Can you work these out from the model? Positions are in its coordinate system, mm. A direction names the side the tool comes from. Give positions to 0.01 mm unless a question says otherwise; leave off trailing zeros. Order: outer loops, then holes, each group sorted by start corner. A loop starts at its lowest first (then second) coordinate and runs counter-clockwise, first axis right, second up. Notation, with made-up numbers: M 36,29 L 95,29 A17 ccw 95,51 Z; hole C 73,10 d2. An arc over 180 degrees is marked long. Use one line per item in the form item = value. Start each with the question number.
1. I want a section at B-B, the plane z = 67. List the corners of the cut face in (x, y) for me, and give its area (3 significant figures).
2. I need wall thicknesses on L1, parallel to Y at x = 4, z = 12; L2, parallel to Y at x = 4, z = 102.5; L3, parallel to Z at x = 22.5, y = 38. Which ranges of each line are inside material? Lowest first, please.
3. For faces 5 (the face through (0, -10, 58)), 6 (the face through (1.479, -7.876, 100.979)), 7 (the face through (-8, 2.96, 103)), which set-ups out of +Z, -Z, +X, -X, +Y, -Y let a thin tool reach every point of the face, with its end or its side?
4. I want a section at A-A, the plane y = 12. List the corners of the cut face in (x, z) for me.
5. Will these pins go through, and if not, where does the flat tip stop? P1, Ø10.5, axis at x = -8, z = 32, coming from the -Y side; P2, Ø2, axis at y = 8.5, z = 49, coming from the -X side; P3, Ø1, axis at y = -2, z = 34.5, coming from the -X side.
6. I want a section at C-C, the plane y = 60.21. List the corners of the cut face in (x, z) for me, and give its area (3 significant figures).
7. I want a section at D-D, the plane x = 14. List the corners of the cut face in (y, z) for me (3 decimals).
8. We'd pull the mould along Z, two halves only. Please class faces 1 (the face through (32.195, 61.697, 1.232)), 2 (the face through (1.48, -7.9, 11.02)), 3 (the face through (14, 24, 0)), 4 (the face through (14, 24, 115)): +Z half, -Z half, draft (parallel to the pull), parting line (faces both ways), or undercut.
```python
from build123d import *

# Parameters (mm, degrees)
SALIENTE_EXTRUIR1_DEPTH = 115
CROQUIS5_W              = 76.000174198
CROQUIS5_H              = 57.319794633
CORTAR_EXTRUIR2_DEPTH   = 16
CROQUIS6_W              = 76.000174198
CROQUIS6_H              = 7.5
CROQUIS6_W_2            = 76
SALIENTE_EXTRUIR2_DEPTH = 10.35
REDONDEO1_R             = 1
CROQUIS7_W              = 115
CROQUIS7_H              = 90
SALIENTE_EXTRUIR3_DEPTH = 5
CROQUIS14_W             = 115
CROQUIS14_H             = 90
CROQUIS14_W_2           = 110
CROQUIS14_H_2           = 85
SALIENTE_EXTRUIR5_DEPTH = 30
CORTAR_EXTRUIR5_REACH   = 26.29
CROQUIS15_R             = 1.8
CORTAR_EXTRUIR6_REACH   = 4.5
CORTAR_EXTRUIR7_DEPTH   = 3
CROQUIS19_R             = 1.5
CORTAR_EXTRUIR8_DEPTH   = 116


with BuildPart() as part:
    # Croquis1 → Saliente-Extruir1 (new body)
    with BuildSketch(Plane.XY):
        with BuildLine():
            Line((0, 49.71), (-16.64, 49.71))
            ThreePointArc((-16.64, 49.71), (-17.347106781, 49.417106781), (-17.64, 48.71))
            Line((-17.64, 48.71), (-17.64, 35.71))
            ThreePointArc((-17.64, 35.71), (-17.347106781, 35.002893219), (-16.64, 34.71))
            Line((-16.64, 34.71), (-16.322634469, 34.71))
            ThreePointArc((-16.322634469, 34.71), (-15.745851008, 34.89310292), (-15.380289019, 35.375358322))
            Line((-15.380289019, 35.375358322), (-14.64, 37.46))
            Line((-14.64, 37.46), (-13.64, 37.46))
            Line((-13.64, 37.46), (-13.64, 3.96))
            ThreePointArc((-13.64, 3.96), (-13.347106781, 3.252893219), (-12.64, 2.96))
            Line((-12.64, 2.96), (-4.22, 2.96))
            ThreePointArc((-4.22, 2.96), (-3.72, 2.46), (-4.22, 1.96))
            Line((-4.22, 1.96), (-14.72, 1.96))
            Line((-14.72, 1.96), (-14.72, 4.12))
            Line((-14.72, 4.12), (-14.839626167, 4.12))
            ThreePointArc((-14.839626167, 4.12), (-15.19514923, 4.054667509), (-15.504217878, 3.867206703))
            Line((-15.504217878, 3.867206703), (-18.954591711, 0.798323834))
            ThreePointArc((-18.954591711, 0.798323834), (-19.202302502, 0.460634096), (-19.29, 0.051117131))
            Line((-19.29, 0.051117131), (-19.29, 0))
            Line((-19.29, 0), (0, 0))
            Line((0, 0), (0, 49.71))
        make_face()
    extrude(amount=SALIENTE_EXTRUIR1_DEPTH)

    # Croquis5 → Cortar-Extruir2 (cut)
    with BuildSketch(Plane.ZY.offset(19.29)):
        with Locations((53, 24.620732186)):
            Rectangle(CROQUIS5_W, CROQUIS5_H)
    extrude(amount=-CORTAR_EXTRUIR2_DEPTH, mode=Mode.SUBTRACT)

    # Croquis6 → Saliente-Extruir2 (add)
    with BuildSketch(Plane.ZY.offset(3.29)):
        with Locations((53, 45.96)):
            Rectangle(CROQUIS6_W, CROQUIS6_H)
        with Locations((52.999912901, 6.71)):
            Rectangle(CROQUIS6_W_2, CROQUIS6_H)
    extrude(amount=SALIENTE_EXTRUIR2_DEPTH)

    # Redondeo1
    redondeo1_edges = [part.edges().sort_by_distance(p)[0] for p in [
        (-13.64, 2.96, 52.999912901),
    ]]
    fillet(redondeo1_edges, radius=REDONDEO1_R)

    # Croquis7 → Saliente-Extruir3 (add)
    with BuildSketch(Plane(origin=(0, 0, 0), x_dir=(0, 0, -1), z_dir=(1, 0, 0))):
        with Locations((-57.5, 24.71)):
            Rectangle(CROQUIS7_W, CROQUIS7_H)
    extrude(amount=SALIENTE_EXTRUIR3_DEPTH)

    # Croquis14 → Saliente-Extruir5 (add)
    with BuildSketch(Plane(origin=(5, 0, 0), x_dir=(0, 0, -1), z_dir=(1, 0, 0))):
        with Locations((-57.5, 24.71)):
            Rectangle(CROQUIS14_W, CROQUIS14_H)
        with Locations((-57.5, 24.71)):
            Rectangle(CROQUIS14_W_2, CROQUIS14_H_2, mode=Mode.SUBTRACT)
    extrude(amount=SALIENTE_EXTRUIR5_DEPTH)

    # Croquis15 → Cortar-Extruir5 (cut, up to next)
    with BuildSketch(Plane(origin=(5, 0, 0), x_dir=(0, 0, -1), z_dir=(1, 0, 0)), mode=Mode.PRIVATE) as cortar_extruir5_sk1:
        with Locations((-102.5, 54.71)):
            Circle(CROQUIS15_R)
    cortar_extruir5_tool1 = extrude(cortar_extruir5_sk1.sketch, amount=-CORTAR_EXTRUIR5_REACH, mode=Mode.PRIVATE) & part.part
    add(cortar_extruir5_tool1.solids().sort_by_distance((5, 54.71, 102.5))[0], mode=Mode.SUBTRACT)
    # Croquis15 → Cortar-Extruir5 (cut, up to next)
    with BuildSketch(Plane(origin=(5, 0, 0), x_dir=(0, 0, -1), z_dir=(1, 0, 0)), mode=Mode.PRIVATE) as cortar_extruir5_sk2:
        with Locations((-102.5, -5.29)):
            Circle(CROQUIS15_R)
    cortar_extruir5_tool2 = extrude(cortar_extruir5_sk2.sketch, amount=-CORTAR_EXTRUIR5_REACH, mode=Mode.PRIVATE) & part.part
    add(cortar_extruir5_tool2.solids().sort_by_distance((5, -5.29, 102.5))[0], mode=Mode.SUBTRACT)
    # Croquis15 → Cortar-Extruir5 (cut, up to next)
    with BuildSketch(Plane(origin=(5, 0, 0), x_dir=(0, 0, -1), z_dir=(1, 0, 0)), mode=Mode.PRIVATE) as cortar_extruir5_sk3:
        with Locations((-12.5, -5.29)):
            Circle(CROQUIS15_R)
    cortar_extruir5_tool3 = extrude(cortar_extruir5_sk3.sketch, amount=-CORTAR_EXTRUIR5_REACH, mode=Mode.PRIVATE) & part.part
    add(cortar_extruir5_tool3.solids().sort_by_distance((5, -5.29, 12.5))[0], mode=Mode.SUBTRACT)
    # Croquis15 → Cortar-Extruir5 (cut, up to next)
    with BuildSketch(Plane(origin=(5, 0, 0), x_dir=(0, 0, -1), z_dir=(1, 0, 0)), mode=Mode.PRIVATE) as cortar_extruir5_sk4:
        with Locations((-12.5, 54.71)):
            Circle(CROQUIS15_R)
    cortar_extruir5_tool4 = extrude(cortar_extruir5_sk4.sketch, amount=-CORTAR_EXTRUIR5_REACH, mode=Mode.PRIVATE) & part.part
    add(cortar_extruir5_tool4.solids().sort_by_distance((5, 54.71, 12.5))[0], mode=Mode.SUBTRACT)

    # Croquis16 → Cortar-Extruir6 (cut, up to next)
    with BuildSketch(Plane(origin=(0, 0, 112.5), x_dir=(-1, 0, 0), z_dir=(0, 0, -1)), mode=Mode.PRIVATE) as cortar_extruir6_sk1:
        with BuildLine():
            Line((-5, -4.415), (-5, 15.585))
            Line((-5, 15.585), (-18, 15.585))
            ThreePointArc((-18, 15.585), (-19.414213562, 14.999213562), (-20, 13.585))
            Line((-20, 13.585), (-20, -2.415))
            ThreePointArc((-20, -2.415), (-19.414213562, -3.829213562), (-18, -4.415))
            Line((-18, -4.415), (-5, -4.415))
        make_face()
    cortar_extruir6_tool1 = extrude(cortar_extruir6_sk1.sketch, amount=-CORTAR_EXTRUIR6_REACH, mode=Mode.PRIVATE) & part.part
    add(cortar_extruir6_tool1.solids().sort_by_distance((12.459404, 5.585, 112.5))[0], mode=Mode.SUBTRACT)

    # Croquis17 → Cortar-Extruir7 (cut)
    with BuildSketch(Plane.ZY):
        Polygon((12.5, 51.245898385), (15.5, 52.977949192), (15.5, 56.442050808), (12.5, 58.174101615), (9.5, 56.442050808), (9.5, 52.977949192), align=None)
        Polygon((9.5, -3.557949192), (12.5, -1.825898385), (15.5, -3.557949192), (15.5, -7.022050808), (12.5, -8.754101615), (9.5, -7.022050808), align=None)
        Polygon((105.5, 52.977949192), (102.5, 51.245898385), (99.5, 52.977949192), (99.5, 56.442050808), (102.5, 58.174101615), (105.5, 56.442050808), align=None)
        Polygon((102.5, -1.825898385), (99.5, -3.557949192), (99.5, -7.022050808), (102.5, -8.754101615), (105.5, -7.022050808), (105.5, -3.557949192), align=None)
    extrude(amount=-CORTAR_EXTRUIR7_DEPTH, mode=Mode.SUBTRACT)

    # Croquis19 → Cortar-Extruir8 (cut, through all)
    with BuildSketch(Plane(origin=(0, 0, 0), x_dir=(-1, 0, 0), z_dir=(0, 0, -1))):
        with Locations((-32, 60.21)):
            Circle(CROQUIS19_R)
    extrude(amount=-CORTAR_EXTRUIR8_DEPTH, mode=Mode.SUBTRACT)


solid = part.part
```
Check result:
q1.outline = M -13.64,3.96 A1 ccw -12.64,2.96 L -3.29,2.96 L -3.29,0 L 0,0 L 0,-20.29 L 35,-20.29 L 35,-17.79 L 5,-17.79 L 5,67.21 L 35,67.21 L 35,69.71 L 0,69.71 L 0,49.71 L -13.64,49.71 L -13.64,42.21 L -3.29,42.21 L -3.29,10.46 L -13.64,10.46 Z
q1.area = 919 mm2
q2.L1 = -20.29 to -7.02, -3.56 to 52.98, 56.44 to 69.71
q2.L2 = -20.29 to -7.09, -3.49 to 52.91, 56.51 to 69.71
q2.L3 = 0 to 2.5, 112.5 to 115
q3.face_5 = +Z, -Z, -X, -Y
q3.face_6 = -X
q3.face_7 = +Z, -Z
q4.outline = M -13.64,0 L 35,0 L 35,2.5 L 5,2.5 L 5,115 L -13.64,115 L -13.64,91 L -3.29,91 L -3.29,15 L -13.64,15 Z; M 20,112.5 L 35,112.5 L 35,115 L 20,115 Z
q5.P1 = 0
q5.P2 = -13.64
q5.P3 = 0
q6.outline = M 0,0 L 30.5,0 L 30.5,2.5 L 5,2.5 L 5,112.5 L 30.5,112.5 L 30.5,115 L 0,115 Z; M 33.5,0 L 35,0 L 35,2.5 L 33.5,2.5 Z; M 33.5,112.5 L 35,112.5 L 35,115 L 33.5,115 Z
q6.area = 710 mm2
q7.outline = M -20.29,0 L 69.71,0 L 69.71,115 L 15.585,115 L 15.585,112.5 L 67.21,112.5 L 67.21,2.5 L -17.79,2.5 L -17.79,112.5 L -4.415,112.5 L -4.415,115 L -20.29,115 Z
q8.face_1 = draft
q8.face_2 = undercut
q8.face_3 = -Z half
q8.face_4 = +Z half
